Build history of the part. All positions in model axes, mm. A direction names the side the tool comes from. Give positions to 0.01 mm unless a question says otherwise; leave off trailing zeros. Loops run counter-clockwise (first coordinate to the right, second up) from the corner with the lowest first, then second, coordinate; pieces in that order, holes last. Notation, with made-up numbers: (42, 67.5) -> (94, 67.5) arc R28 cw to (94, 101.5) -> close; hole circle Ø11 at (49, 81). An arc over 180 degrees is marked (long way). One line per question, with ' | ' between items. Start each with the question number.
(1) Drill centre lines: L1, parallel to X at y = 2.25, z = -32.5; L2, parallel to X at y = -1, z = -32.5; L3, parallel to X at y = -2, z = -37.5. Where is each one in solid material? Low to high. Write a range as from..to.
(2) Flat gauge pins, fed straight in: pin 1 Ø3 at (x, y) = (-101, -3.5) entering from +Z; pin 2 Ø1.5 at (y, z) = (-2.5, -30.5) entering from +X; pin 3 Ø1.5 at (x, y) = (-64.5, -3.5) entering from -Z. Where does each tip first touch, or does it go through?
(3) Mould opens along Z. For faces 5 (the face through (-65, -5, -32)), 6 (the face through (-65, 2, 0)), 7 (the face through (-66.206, 0.07, -30.081)), 8 (the face through (-65, 2, -65)) say: pulls with the +Z half, pulls with the -Z half, needs draft (parallel to the pull), parting line crosses it, or undercut.
(4) Slice it at D-D, the plane x = -93.5. Write the cut outline in (y, z), then the cut area to 3 significant figures.
(5) Slice it at B-B, the plane z = -22. Write the cut outline in (x, y), then the cut area to 3 significant figures.
(6) Slice it at A-A, the plane x = -70. Write the cut outline in (y, z), then the cut area to 3 significant figures.
(7) 3-axis set-ups, long thin cutter, end or side, ignore diameter. For faces 1 (the face through (-123.18, -2, -33)), 2 (the face through (-5.1, -2, -33)), 3 (the face through (-65, -2, -59.9)), 4 (the face through (-65, -2, -5.1)): which of +Z, -Z, +X, -X, +Y, -Y reach the whole face in a straight line?
(8) Slice it at C-C, the plane z = -32.5. Write the cut outline in (x, y), then the cut area to 3 significant figures.
```python
from build123d import *

# Parameters (mm, degrees)
SKETCH1_W           = 128.28
SKETCH1_H           = 65
BOSS_EXTRUDE1_DEPTH = 5
SKETCH3_W           = 118.08
SKETCH3_H           = 54.8
BOSS_EXTRUDE2_DEPTH = 5
CUT_EXTRUDE1_REACH  = 146.155
SKETCH4_R           = 4.5


with BuildPart() as part:
    # Sketch1 → Boss-Extrude1 (new body)
    with BuildSketch(Plane(origin=(0, 0, 0), x_dir=(1, 0, 0), z_dir=(0, 1, 0))):
        with Locations((-64.14, 32.5)):
            Rectangle(SKETCH1_W, SKETCH1_H)
    extrude(amount=BOSS_EXTRUDE1_DEPTH)

    # Sketch3 → Boss-Extrude2 (add)
    with BuildSketch(Plane.XZ):
        with Locations((-64.14, -32.5)):
            Rectangle(SKETCH3_W, SKETCH3_H)
    extrude(amount=BOSS_EXTRUDE2_DEPTH)

    # Sketch4 → Cut-Extrude1 (cut, up to next)
    with BuildSketch(Plane(origin=(0, 5, 0), x_dir=(1, 0, 0), z_dir=(0, 1, 0)), mode=Mode.PRIVATE) as cut_extrude1_sk1:
        with Locations(Location((-70, 32.5, 0), (0, 0, 270))):
            Circle(SKETCH4_R)
    cut_extrude1_tool1 = extrude(cut_extrude1_sk1.sketch, amount=-CUT_EXTRUDE1_REACH, mode=Mode.PRIVATE) & part.part
    add(cut_extrude1_tool1.solids().sort_by_distance((-70, 5, -32.5))[0], mode=Mode.SUBTRACT)


solid = part.part
```
Final values:
1) L1: -128.28..-74.5, -65.5..0 | L2: -123.18..-74.5, -65.5..-5.1 | L3: -123.18..-5.1
2) pin 1: z = -5.1 | pin 2: x = -5.1 | pin 3: z = -59.9
3) face 5: needs draft | face 6: pulls with the +Z half | face 7: undercut | face 8: pulls with the -Z half
4) outline: (-5, -59.9) -> (0, -59.9) -> (0, -65) -> (5, -65) -> (5, 0) -> (0, 0) -> (0, -5.1) -> (-5, -5.1) -> close | area: 599 mm2
5) outline: (-128.28, 0) -> (-123.18, 0) -> (-123.18, -5) -> (-5.1, -5) -> (-5.1, 0) -> (0, 0) -> (0, 5) -> (-128.28, 5) -> close | area: 1,230 mm2
6) outline: (-5, -59.9) -> (0, -59.9) -> (0, -65) -> (5, -65) -> (5, -37) -> (-5, -37) -> close; (-5, -28) -> (5, -28) -> (5, 0) -> (0, 0) -> (0, -5.1) -> (-5, -5.1) -> close | area: 509 mm2
7) face 1: +Z, -Z, -X, -Y | face 2: +Z, -Z, +X, -Y | face 3: -Z, +X, -X, -Y | face 4: +Z, +X, -X, -Y
8) outline: (-128.28, 0) -> (-123.18, 0) -> (-123.18, -5) -> (-74.5, -5) -> (-74.5, 5) -> (-128.28, 5) -> close; (-65.5, -5) -> (-5.1, -5) -> (-5.1, 0) -> (0, 0) -> (0, 5) -> (-65.5, 5) -> close | area: 1,140 mm2
